```python
from build123d import *

# Parameters (mm, degrees)
SKETCH1_R           = 1.6
BOSS_EXTRUDE1_DEPTH = 3


with BuildPart() as part:
    # Sketch1 → Boss-Extrude1 (new body)
    with BuildSketch(Plane(origin=(0, 0, 0), x_dir=(1, 0, 0), z_dir=(0, 1, 0))):
        with BuildLine():
            Line((-70, 42.5), (70, 42.5))
            ThreePointArc((70, 42.5), (73.535533906, 41.035533906), (75, 37.5))
            Line((75, 37.5), (75, -37.5))
            ThreePointArc((75, -37.5), (73.535533906, -41.035533906), (70, -42.5))
            Line((70, -42.5), (-70, -42.5))
            ThreePointArc((-70, -42.5), (-73.535533906, -41.035533906), (-75, -37.5))
            Line((-75, -37.5), (-75, 37.5))
            ThreePointArc((-75, 37.5), (-73.535533906, 41.035533906), (-70, 42.5))
        make_face()
        with Locations(Location((13.25, 21.25, 0), (0, 0, 270))):
            Circle(SKETCH1_R, mode=Mode.SUBTRACT)
        with Locations(Location((-70, 37.5, 0), (0, 0, 270))):
            Circle(SKETCH1_R, mode=Mode.SUBTRACT)
        with Locations(Location((-70, -37.5, 0), (0, 0, 90))):
            Circle(SKETCH1_R, mode=Mode.SUBTRACT)
        with Locations(Location((70, -37.5, 0), (0, 0, 270))):
            Circle(SKETCH1_R, mode=Mode.SUBTRACT)
        with Locations(Location((70, 37.5, 0), (0, 0, 90))):
            Circle(SKETCH1_R, mode=Mode.SUBTRACT)
        with Locations(Location((61.75, 21.25, 0), (0, 0, 270))):
            Circle(SKETCH1_R, mode=Mode.SUBTRACT)
        with Locations(Location((13.25, -21.25, 0), (0, 0, 90))):
            Circle(SKETCH1_R, mode=Mode.SUBTRACT)
        with Locations(Location((61.75, -21.25, 0), (0, 0, 90))):
            Circle(SKETCH1_R, mode=Mode.SUBTRACT)
        with Locations(Location((-34.65, 27.81, 0), (0, 0, 270))):
            Circle(SKETCH1_R, mode=Mode.SUBTRACT)
        with Locations(Location((-34.65, -27.81, 0), (0, 0, 90))):
            Circle(SKETCH1_R, mode=Mode.SUBTRACT)
        with Locations(Location((-15.35, -27.81, 0), (0, 0, 270))):
            Circle(SKETCH1_R, mode=Mode.SUBTRACT)
        with Locations(Location((-15.35, 27.81, 0), (0, 0, 90))):
            Circle(SKETCH1_R, mode=Mode.SUBTRACT)
        with Locations(Location((-41.5, 38.5, 0), (0, 0, 270))):
            Circle(SKETCH1_R, mode=Mode.SUBTRACT)
        with Locations(Location((-41.5, -38.5, 0), (0, 0, 90))):
            Circle(SKETCH1_R, mode=Mode.SUBTRACT)
        with Locations(Location((41.5, -38.5, 0), (0, 0, 270))):
            Circle(SKETCH1_R, mode=Mode.SUBTRACT)
        with Locations(Location((41.5, 38.5, 0), (0, 0, 90))):
            Circle(SKETCH1_R, mode=Mode.SUBTRACT)
        with Locations(Location((-68.96, 5.46, 0), (0, 0, 270))):
            Circle(SKETCH1_R, mode=Mode.SUBTRACT)
        with BuildLine():
            Line((10.75, 17.5), (15.75, 17.5))
            ThreePointArc((15.75, 17.5), (17.164213562, 16.914213562), (17.75, 15.5))
            Line((17.75, 15.5), (17.75, -15.5))
            ThreePointArc((17.75, -15.5), (17.164213562, -16.914213562), (15.75, -17.5))
            Line((15.75, -17.5), (10.75, -17.5))
            ThreePointArc((10.75, -17.5), (9.335786438, -16.914213562), (8.75, -15.5))
            Line((8.75, -15.5), (8.75, 15.5))
            ThreePointArc((8.75, 15.5), (9.335786438, 16.914213562), (10.75, 17.5))
        make_face(mode=Mode.SUBTRACT)
        with BuildLine():
            Line((64.25, -17.5), (59.25, -17.5))
            ThreePointArc((59.25, -17.5), (57.835786438, -16.914213562), (57.25, -15.5))
            Line((57.25, -15.5), (57.25, 15.5))
            ThreePointArc((57.25, 15.5), (57.835786438, 16.914213562), (59.25, 17.5))
            Line((59.25, 17.5), (64.25, 17.5))
            ThreePointArc((64.25, 17.5), (65.664213562, 16.914213562), (66.25, 15.5))
            Line((66.25, 15.5), (66.25, -15.5))
            ThreePointArc((66.25, -15.5), (65.664213562, -16.914213562), (64.25, -17.5))
        make_face(mode=Mode.SUBTRACT)
        with BuildLine():
            Line((-58.54, 7.06), (-49.54, 7.06))
            ThreePointArc((-49.54, 7.06), (-47.94, 5.46), (-49.54, 3.86))
            Line((-49.54, 3.86), (-58.54, 3.86))
            ThreePointArc((-58.54, 3.86), (-60.14, 5.46), (-58.54, 7.06))
        make_face(mode=Mode.SUBTRACT)
        with BuildLine():
            Line((-64.05, -34.5), (-58.95, -34.5))
            ThreePointArc((-58.95, -34.5), (-57.535786438, -33.914213562), (-56.95, -32.5))
            Line((-56.95, -32.5), (-56.95, -22.5))
            ThreePointArc((-56.95, -22.5), (-57.535786438, -21.085786438), (-58.95, -20.5))
            Line((-58.95, -20.5), (-64.05, -20.5))
            ThreePointArc((-64.05, -20.5), (-65.464213562, -21.085786438), (-66.05, -22.5))
            Line((-66.05, -22.5), (-66.05, -32.5))
            ThreePointArc((-66.05, -32.5), (-65.464213562, -33.914213562), (-64.05, -34.5))
        make_face(mode=Mode.SUBTRACT)
        with BuildLine():
            Line((-64.05, 34.5), (-58.95, 34.5))
            ThreePointArc((-58.95, 34.5), (-57.535786438, 33.914213562), (-56.95, 32.5))
            Line((-56.95, 32.5), (-56.95, 22.5))
            ThreePointArc((-56.95, 22.5), (-57.535786438, 21.085786438), (-58.95, 20.5))
            Line((-58.95, 20.5), (-64.05, 20.5))
            ThreePointArc((-64.05, 20.5), (-65.464213562, 21.085786438), (-66.05, 22.5))
            Line((-66.05, 22.5), (-66.05, 32.5))
            ThreePointArc((-66.05, 32.5), (-65.464213562, 33.914213562), (-64.05, 34.5))
        make_face(mode=Mode.SUBTRACT)
        with BuildLine():
            Line((53.520093719, -34.5), (64.479906281, -34.5))
            ThreePointArc((64.479906281, -34.5), (65.908328248, -33.908328248), (66.5, -32.479906281))
            Line((66.5, -32.479906281), (66.5, -28.520093719))
            ThreePointArc((66.5, -28.520093719), (65.908328248, -27.091671752), (64.479906281, -26.5))
            Line((64.479906281, -26.5), (53.520093719, -26.5))
            ThreePointArc((53.520093719, -26.5), (52.091671752, -27.091671752), (51.5, -28.520093719))
            Line((51.5, -28.520093719), (51.5, -32.479906281))
            ThreePointArc((51.5, -32.479906281), (52.091671752, -33.908328248), (53.520093719, -34.5))
        make_face(mode=Mode.SUBTRACT)
        with BuildLine():
            Line((53.520093719, 34.5), (64.479906281, 34.5))
            ThreePointArc((64.479906281, 34.5), (65.908328248, 33.908328248), (66.5, 32.479906281))
            Line((66.5, 32.479906281), (66.5, 28.520093719))
            ThreePointArc((66.5, 28.520093719), (65.908328248, 27.091671752), (64.479906281, 26.5))
            Line((64.479906281, 26.5), (53.520093719, 26.5))
            ThreePointArc((53.520093719, 26.5), (52.091671752, 27.091671752), (51.5, 28.520093719))
            Line((51.5, 28.520093719), (51.5, 32.479906281))
            ThreePointArc((51.5, 32.479906281), (52.091671752, 33.908328248), (53.520093719, 34.5))
        make_face(mode=Mode.SUBTRACT)
        with BuildLine():
            Line((-7.5, -20.979906281), (-7.5, -19.020093719))
            ThreePointArc((-7.5, -19.020093719), (-8.091671752, -17.591671752), (-9.520093719, -17))
            Line((-9.520093719, -17), (-40.479906281, -17))
            ThreePointArc((-40.479906281, -17), (-41.908328248, -17.591671752), (-42.5, -19.020093719))
            Line((-42.5, -19.020093719), (-42.5, -20.979906281))
            ThreePointArc((-42.5, -20.979906281), (-41.908328248, -22.408328248), (-40.479906281, -23))
            Line((-40.479906281, -23), (-9.520093719, -23))
            ThreePointArc((-9.520093719, -23), (-8.091671752, -22.408328248), (-7.5, -20.979906281))
        make_face(mode=Mode.SUBTRACT)
        with BuildLine():
            Line((-40.479906281, 23), (-9.520093719, 23))
            ThreePointArc((-9.520093719, 23), (-8.091671752, 22.408328248), (-7.5, 20.979906281))
            Line((-7.5, 20.979906281), (-7.5, 19.020093719))
            ThreePointArc((-7.5, 19.020093719), (-8.091671752, 17.591671752), (-9.520093719, 17))
            Line((-9.520093719, 17), (-40.479906281, 17))
            ThreePointArc((-40.479906281, 17), (-41.908328248, 17.591671752), (-42.5, 19.020093719))
            Line((-42.5, 19.020093719), (-42.5, 20.979906281))
            ThreePointArc((-42.5, 20.979906281), (-41.908328248, 22.408328248), (-40.479906281, 23))
        make_face(mode=Mode.SUBTRACT)
    extrude(amount=BOSS_EXTRUDE1_DEPTH)


solid = part.part
```
The model under review builds one solid part; all positions refer to its coordinate system, in mm. A direction names the side the tool comes from. Round coordinates to 2 decimals unless told otherwise and drop trailing zeros. Loops run counter-clockwise (first coordinate to the right, second up) from the corner with the lowest first, then second, coordinate; pieces in that order, holes last. Notation, with made-up numbers: (58, -28.5) - (72, -28.5) arc R21 cw to (72, -9.5) - close; hole circle Ø10 at (-33.75, -20). An arc over 180 degrees is marked (long way). Use a Markdown table: item, result. Add a question column.
Q1. Machinability: for faces 1 (the face through (-25, 1, 17)), 2 (the face through (73.57, 1.48, 41)), which of the approach directions +Z, -Z, +X, -X, +Y, -Y give a long, thin tool a straight path to every point of the face, cutting with its end or side? Answer none if there is none.
Q2. For probe 1 along Z at (x, y) = (54.5, 1.8); probe 2 along Z at (x, y) = (64, 2.05); probe 3 along Z at (x, y) = (-22, 1.35), list the stretches that pass through material, from the lowest coordinate up.
Q3. Add section B-B (z = -2). State the section outline as (x, y) points, plus the area to 3 significant figures.
Q4. Add section C-C (x = 41.5). State the section outline as (y, z) points.
Q5. Add section D-D (z = -24.5). State the section outline as (x, y) points, plus the area to 3 significant figures.
Q6. Add section A-A (x = 61.75). State the section outline as (y, z) points.
Q7. The part is to be moulded in two halves that separate along Z. For faces 3 (the face through (1, 1, 42.5)), 4 (the face through (66.25, 1, 0)), 5 (the face through (-61, 1, 20.5)), say which applies: pulls with the +Z half, pulls with the -Z half, needs draft (parallel to the pull), parting line crosses it, or undercut.
Worked answers:
| question | item | result |
|---|---|---|
| 1 | face 1 | +Y, -Y |
| 1 | face 2 | +Z, +X, +Y, -Y |
| 2 | probe 1 | -42.5 to -34.5, -26.5 to 26.5, 34.5 to 42.5 |
| 2 | probe 2 | -42.5 to -34.5, -26.5 to -17.5, 17.5 to 26.5, 34.5 to 42.5 |
| 2 | probe 3 | -42.5 to -23, -17 to 17, 23 to 42.5 |
| 3 | outline | (-75, 0) - (8.75, 0) - (8.75, 3) - (-75, 3) - close; (17.75, 0) - (57.25, 0) - (57.25, 3) - (17.75, 3) - close; (66.25, 0) - (75, 0) - (75, 3) - (66.25, 3) - close |
| 3 | area | 396 mm² |
| 4 | outline | (0, -42.5) - (3, -42.5) - (3, -40.1) - (0, -40.1) - close; (0, -36.9) - (3, -36.9) - (3, 36.9) - (0, 36.9) - close; (0, 40.1) - (3, 40.1) - (3, 42.5) - (0, 42.5) - close |
| 5 | outline | (-75, 0) - (-66.05, 0) - (-66.05, 3) - (-75, 3) - close; (-56.95, 0) - (75, 0) - (75, 3) - (-56.95, 3) - close |
| 5 | area | 423 mm² |
| 6 | outline | (0, -42.5) - (3, -42.5) - (3, -34.5) - (0, -34.5) - close; (0, -26.5) - (3, -26.5) - (3, -22.85) - (0, -22.85) - close; (0, -19.65) - (3, -19.65) - (3, -17.5) - (0, -17.5) - close; (0, 17.5) - (3, 17.5) - (3, 19.65) - (0, 19.65) - close; (0, 22.85) - (3, 22.85) - (3, 26.5) - (0, 26.5) - close; (0, 34.5) - (3, 34.5) - (3, 42.5) - (0, 42.5) - close |
| 7 | face 3 | pulls with the +Z half |
| 7 | face 4 | undercut |
| 7 | face 5 | undercut |
